Source: CAD feature listing. Evaluate the final solid. Frame: model axes, mm. Give positions to 0.01 mm unless a question says otherwise; leave off trailing zeros. Write each loop counter-clockwise with the first axis right and the second up, starting at its lowest first coordinate (ties: lowest second). Pieces come first, ordered by that corner, then holes.
```python
from build123d import *

# Parameters (mm, degrees)
ESQUISSE1_W             = 444.3
ESQUISSE1_H             = 51.18
BOSS_EXTRU_1_DEPTH      = 3
ESQUISSE2_R             = 2.6
ENL_V_MAT_EXTRU_1_DEPTH = 20
ESQUISSE3_W             = 69
ESQUISSE3_H             = 3
ENL_V_MAT_EXTRU_2_DEPTH = 11


with BuildPart() as part:
    # Esquisse1 → Boss.-Extru.1 (new body)
    with BuildSketch(Plane.XY):
        with Locations((-222.15, 25.59)):
            Rectangle(ESQUISSE1_W, ESQUISSE1_H)
    extrude(amount=BOSS_EXTRU_1_DEPTH)

    # Esquisse2 → Enlèv. mat.-Extru.1 (cut)
    with BuildSketch(Plane.XY.offset(3)):
        with Locations((-13, 43.165806832)):
            Circle(ESQUISSE2_R)
        with Locations((-431.3, 40.774785784)):
            Circle(ESQUISSE2_R)
    extrude(amount=-ENL_V_MAT_EXTRU_1_DEPTH, mode=Mode.SUBTRACT)

    # Esquisse3 → Enlèv. mat.-Extru.2 (cut)
    with BuildSketch(Plane.XZ):
        with Locations((-397.3, 1.5)):
            Rectangle(ESQUISSE3_W, ESQUISSE3_H)
        with Locations((-47, 1.5)):
            Rectangle(ESQUISSE3_W, ESQUISSE3_H)
    extrude(amount=-ENL_V_MAT_EXTRU_2_DEPTH, mode=Mode.SUBTRACT)


solid = part.part
```
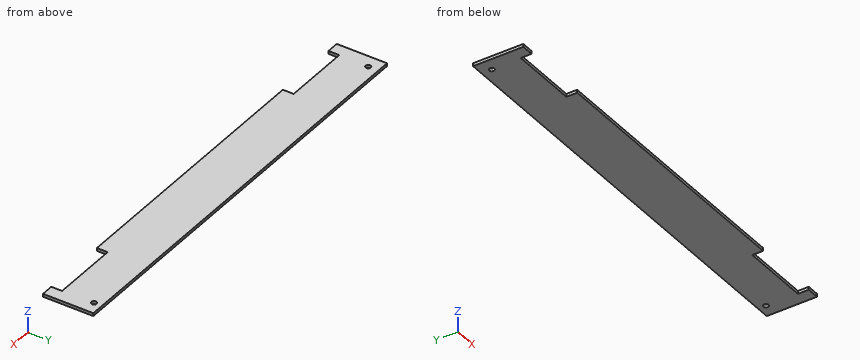
1. Line query: probe 1 along X at (y, z) = (6, 1); probe 2 along Y at (x, z) = (-13, 2.2); probe 3 along Y at (x, z) = (-431.3, 1.6). Output: solid intervals per line, ascending.
2. Pin query (flat end, axial travel): P1, Ø3, axis at x = -431.3, y = 40.77, coming from the +Z side; P2, Ø1.5, axis at x = -407, z = 1.5, coming from the -Y side. Return the tip coordinate at first contact, or that it passes through.
3. Section query A-A (y = 5). Return loops of the section in (x, z).
4. Section query B-B (z = 0.55). Return loops of the section in (x, y).
The answers:
1. probe 1: x = -444.3 to -431.8, -362.8 to -81.5, -12.5 to 0
1. probe 2: y = 11 to 40.57, 45.77 to 51.18
1. probe 3: y = 11 to 38.17, 43.37 to 51.18
2. P1: passes through
2. P2: stops at y = 11
3. outline: (-444.3, 0) - (-431.8, 0) - (-431.8, 3) - (-444.3, 3) - close; (-362.8, 0) - (-81.5, 0) - (-81.5, 3) - (-362.8, 3) - close; (-12.5, 0) - (0, 0) - (0, 3) - (-12.5, 3) - close
4. outline: (-444.3, 0) - (-431.8, 0) - (-431.8, 11) - (-362.8, 11) - (-362.8, 0) - (-81.5, 0) - (-81.5, 11) - (-12.5, 11) - (-12.5, 0) - (0, 0) - (0, 51.18) - (-444.3, 51.18) - close; hole circle Ø5.2 at (-431.3, 40.77); hole circle Ø5.2 at (-13, 43.17)
